Input: dimensioned drawing with shaded views. Units: mm. Origin: part minimum x, y, z. A direction names the side the tool comes from. Coordinates: 2 decimals unless noted, no trailing zeros. Write each loop counter-clockwise with the first axis right and the second up, starting at its lowest first coordinate (ties: lowest second). Pieces come first, ordered by that corner, then holes. Notation, with made-up numbers: (-38.5, 48.25) -> (-29.5, 48.25) arc R10 cw to (-29.5, 54.25) -> close; hole circle Ø8 at (67, -29.75). An arc over 180 degrees is marked (long way). One line per item, written item: value. Start each with the question number.
1. Section query D-D, the plane x = 8.5. Output: boundary loops of the cut face in (y, z).
2. Section query B-B, the plane y = 10.75. Output: boundary loops of the cut face in (x, z) (1 decimal).
3. Mould query, pull axis Y, two halves, no side actions, for the marked faces 3, 4, 5 and 6. Classes: released by +Y, released by -Y, zero draft, split by the parting line, or undercut.
4. Line query: line 1 (Z direction, x = 14.5, y = 9.5); line 2 (Y direction, x = 16.45, z = 9); line 3 (X direction, y = 12.25, z = 14.5). Output: solid intervals per line, ascending.
5. First-contact query: P1, Ø8, axis at x = 11.5, z = 9, coming from the +Y side; P2, Ø7, axis at y = 7.5, z = 11.5, coming from the -X side; P3, Ø4, axis at y = 4.5, z = 3, coming from the -X side; P4, Ø2.5, axis at x = 8.94, z = 9, coming from the -Y side. Flat tips, straight axial feed; report the tip coordinate or a pass-through.
6. Section query C-C, the plane z = 14. Output: boundary loops of the cut face in (x, y).
7. Access query for the marked faces 1 and 2. Directions: +Z, -Z, +X, -X, +Y, -Y. A direction counts if a zero-diameter tool reaches every point of the face in a straight line with its end or side. Return the directions, or none.
8. Section query A-A, the plane z = 9. Output: boundary loops of the cut face in (x, y).
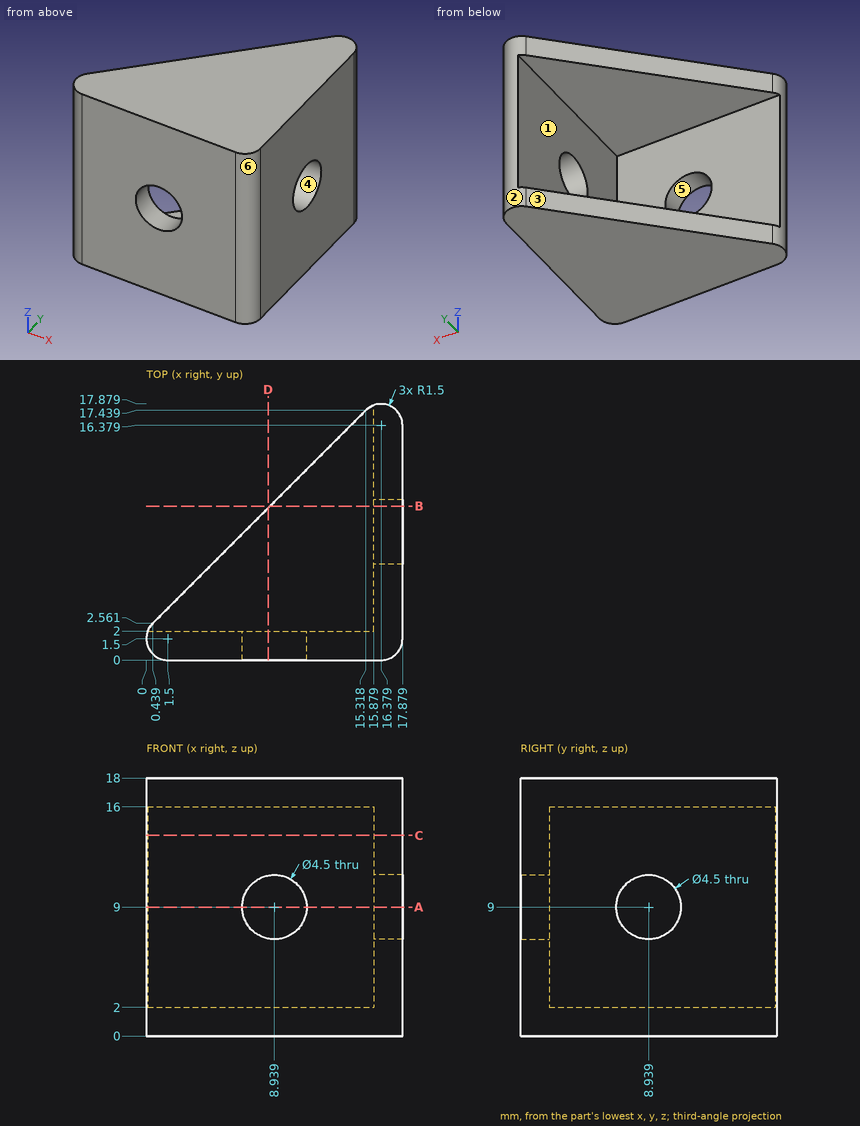
Computed values:
1. outline: (0, 0) -> (10.62, 0) -> (10.62, 2) -> (2, 2) -> (2, 6.79) -> (0, 6.79) -> close; (0, 11.21) -> (2, 11.21) -> (2, 16) -> (10.62, 16) -> (10.62, 18) -> (0, 18) -> close
2. outline: (8.6, 0) -> (17.9, 0) -> (17.9, 7.7) -> (15.9, 7.7) -> (15.9, 2) -> (8.6, 2) -> close; (8.6, 16) -> (15.9, 16) -> (15.9, 10.3) -> (17.9, 10.3) -> (17.9, 18) -> (8.6, 18) -> close
3. face 3: released by +Y
3. face 4: undercut
3. face 5: zero draft
3. face 6: released by -Y
4. line 1: z = 0 to 2, 16 to 18
4. line 2: y = 0 to 6.69, 11.19 to 17.88
4. line 3: x = 15.88 to 17.88
5. P1: stops at y = 2
5. P2: stops at x = 15.88
5. P3: stops at x = 0.65
5. P4: passes through
6. outline: (0.09, 2) arc R1.5 ccw to (1.5, 0) -> (16.38, 0) arc R1.5 ccw to (17.88, 1.5) -> (17.88, 16.38) arc R1.5 ccw to (15.88, 17.79) -> (15.88, 2) -> close
7. face 1: -X, +Y
7. face 2: +Z, -Z, +Y
8. outline: (0.09, 2) arc R1.5 ccw to (1.5, 0) -> (6.69, 0) -> (6.69, 2) -> close; (11.19, 0) -> (16.38, 0) arc R1.5 ccw to (17.88, 1.5) -> (17.88, 6.69) -> (15.88, 6.69) -> (15.88, 2) -> (11.19, 2) -> close; (15.88, 11.19) -> (17.88, 11.19) -> (17.88, 16.38) arc R1.5 ccw to (15.88, 17.79) -> close
